Here's how the part is built. I have some questions about the finished solid (model axes, mm). Give positions to 0.01 mm unless a question says otherwise; leave off trailing zeros. Loops run counter-clockwise (first coordinate to the right, second up) from the corner with the lowest first, then second, coordinate; pieces in that order, holes last.
Q1. Suppose I cut it at C-C (z = 0.25). List the corners of the cut face in (x, y) for me, and give its area (3 significant figures).
Q2. Suppose I cut it at B-B (x = 1.9). List the corners of the cut face in (y, z) for me.
Q3. Suppose I cut it at A-A (y = 4). List the corners of the cut face in (x, z) for me.
Q4. Suppose I cut it at D-D (y = 5). List the corners of the cut face in (x, z) for me.
Q5. Thinking about a two-plate mould opening in Y: for faces 1 (the face through (1.5, -0.048, 0.4)), 2 (the face through (2.783, 3.31, 0.444)), 3 (the face through (1.385, 6.214, 0.444)), which applies, pulls with the +Y half, pulls with the -Y half, needs draft (parallel to the pull), parting line crosses it, or undercut?
Q6. I need wall thicknesses on probe 1 along Y at (x, z) = (1.5, 0.4); probe 2 along Y at (x, z) = (1.75, 0.55); probe 3 along X at (y, z) = (5.5, 0.5). Which ranges of each line are inside material? Lowest first, please.
```python
from build123d import *

# Parameters (mm, degrees)
SKETCH1_R           = 0.5
BOSS_EXTRUDE1_DEPTH = 0.899922


with BuildPart() as part:
    # Sketch1 → Boss-Extrude1 (new body)
    with BuildSketch(Plane.XY):
        with BuildLine():
            Line((1.569871125, 7.70179743), (1.41624751, 7.70179743))
            ThreePointArc((1.41624751, 7.70179743), (0.731524296, 7.430600641), (0.418190556, 6.764105671))
            Line((0.418190556, 6.764105671), (-0.007098742, -0.04820257))
            Line((-0.007098742, -0.04820257), (2.992901258, -0.04820257))
            Line((2.992901258, -0.04820257), (2.567930958, 6.764059536))
            ThreePointArc((2.567930958, 6.764059536), (2.254611183, 7.430584816), (1.569871125, 7.70179743))
        make_face()
        with Locations((1.492901258, 3.70179743)):
            Circle(SKETCH1_R, mode=Mode.SUBTRACT)
        with Locations((1.492901258, 5.20179743)):
            Circle(SKETCH1_R, mode=Mode.SUBTRACT)
        with Locations((1.492901258, 6.70179743)):
            Circle(SKETCH1_R, mode=Mode.SUBTRACT)
    extrude(amount=BOSS_EXTRUDE1_DEPTH)


solid = part.part
```
Solutions:
1. outline: (-0.01, -0.05) - (2.99, -0.05) - (2.57, 6.76) arc R1 ccw to (1.57, 7.7) - (1.42, 7.7) arc R1 ccw to (0.42, 6.76) - close; hole circle Ø1 at (1.49, 3.7); hole circle Ø1 at (1.49, 5.2); hole circle Ø1 at (1.49, 6.7)
1. area: 16.8 mm2
2. outline: (-0.05, 0) - (3.41, 0) - (3.41, 0.9) - (-0.05, 0.9) - close; (3.99, 0) - (4.91, 0) - (4.91, 0.9) - (3.99, 0.9) - close; (5.49, 0) - (6.41, 0) - (6.41, 0.9) - (5.49, 0.9) - close; (6.99, 0) - (7.65, 0) - (7.65, 0.9) - (6.99, 0.9) - close
3. outline: (0.25, 0) - (1.09, 0) - (1.09, 0.9) - (0.25, 0.9) - close; (1.89, 0) - (2.74, 0) - (2.74, 0.9) - (1.89, 0.9) - close
4. outline: (0.31, 0) - (1.04, 0) - (1.04, 0.9) - (0.31, 0.9) - close; (1.95, 0) - (2.68, 0) - (2.68, 0.9) - (1.95, 0.9) - close
5. face 1: pulls with the -Y half
5. face 2: pulls with the +Y half
5. face 3: undercut
6. probe 1: y = -0.05 to 3.2, 4.2 to 4.7, 5.7 to 6.2, 7.2 to 7.7
6. probe 2: y = -0.05 to 3.27, 4.13 to 4.77, 5.63 to 6.27, 7.13 to 7.69
6. probe 3: x = 0.34 to 1.09, 1.89 to 2.65
